from build123d import *

# Parameters (mm, degrees)
SKETCH1_W           = 50.8
SKETCH1_H           = 50.8
BOSS_EXTRUDE1_DEPTH = 2.54
SKETCH2_W           = 50.8
SKETCH2_H           = 50.8
SKETCH2_W_2         = 45.72
SKETCH2_H_2         = 22.86
BOSS_EXTRUDE2_DEPTH = 25.4
SKETCH3_W           = 50.8
SKETCH3_H           = 10.16
CUT_EXTRUDE1_DEPTH  = 25.4


with BuildPart() as part:
    # Sketch1 → Boss-Extrude1 (new body)
    with BuildSketch(Plane(origin=(0, 0, 0), x_dir=(1, 0, 0), z_dir=(0, 1, 0))):
        with Locations((25.4, 25.4)):
            Rectangle(SKETCH1_W, SKETCH1_H)
    extrude(amount=BOSS_EXTRUDE1_DEPTH)

    # Sketch2 → Boss-Extrude2 (add)
    with BuildSketch(Plane(origin=(0, 2.54, 0), x_dir=(1, 0, 0), z_dir=(0, 1, 0))):
        with Locations((25.4, 25.4)):
            Rectangle(SKETCH2_W, SKETCH2_H)
        with Locations((25.4, 25.4)):
            Rectangle(SKETCH2_W_2, SKETCH2_H_2, mode=Mode.SUBTRACT)
    extrude(amount=BOSS_EXTRUDE2_DEPTH)

    # Sketch3 → Cut-Extrude1 (cut)
    with BuildSketch(Plane(origin=(0, 27.94, 0), x_dir=(1, 0, 0), z_dir=(0, 1, 0))):
        with Locations((25.4, 45.72)):
            Rectangle(SKETCH3_W, SKETCH3_H)
        with Locations((25.4, 5.08)):
            Rectangle(SKETCH3_W, SKETCH3_H)
    extrude(amount=-CUT_EXTRUDE1_DEPTH, mode=Mode.SUBTRACT)


solid = part.part
CAD build for the part. Positions are in the model's coordinates, mm. A direction names the side the tool comes from. Round coordinates to 2 decimals unless told otherwise and drop trailing zeros. Write each loop counter-clockwise with the first axis right and the second up, starting at its lowest first coordinate (ties: lowest second). Pieces come first, ordered by that corner, then holes. Notation, with made-up numbers: M 27,47 L 43,47 A12 cw 43,63 Z; hole C 89.25,-12 d1. An arc over 180 degrees is marked long. Put each result on its own line as item: value. Start each with the question number.
1) 3-axis set-ups, long thin cutter, end or side, ignore diameter. For faces 4 (the flat face through (23, 27.94, -13)), 5 (the flat face through (25, 15, -10.16)), 6 (the flat face through (25, 15, -40.64)), 7 (the flat face through (25, 1, 0)), 8 (the flat face through (25, 15, -36.83)): which of +Z, -Z, +X, -X, +Y, -Y reach the whole face in a straight line?
2) Pin check, flat tips, straight feed: pin 1 Ø12.5 at (x, y) = (36.5, 19) entering from -Z; pin 2 Ø8 at (x, z) = (35, -3.5) entering from +Y; pin 3 Ø3 at (x, y) = (26, 14.5) entering from +Z. Stop position of each tip, or through.
3) Pull direction Z, two halves, no side cores. Call faces 1 (the flat face through (25, 2.54, -46)), 2 (the flat face through (25, 1, -50.8)), 3 (the flat face through (48.26, 15, -25)): pulls with the +Z half, pulls with the -Z half, needs draft (parallel to the pull), parting line crosses it, or undercut.
4) Drill centre lines: probe 1 along X at (y, z) = (6.5, -32.5); probe 2 along Z at (x, y) = (20, 19.75); probe 3 along Y at (x, z) = (21.5, -48). Where is each one in solid material? Low to high. Write a range as [from, to].
5) Saw through at D-D, the plane z = -6.5. Write the cut outline in (x, y), and give its area (3 significant figures).
6) Saw through at C-C, the plane y = 18.25. Write the cut outline in (x, z).
7) Saw through at A-A, the plane x = 30. Write the cut outline in (y, z).
8) Saw through at B-B, the plane z = -33. Write the cut outline in (x, y), and give its area (3 significant figures).
Resolved:
1. face 4: +Z, -Z, +X, -X, +Y
1. face 5: +Z, +X, -X, +Y
1. face 6: -Z, +X, -X, +Y
1. face 7: +Z, +X, -X, +Y, -Y
1. face 8: +Y
2. pin 1: z = -40.64
2. pin 2: y = 2.54
2. pin 3: z = -10.16
3. face 1: needs draft
3. face 2: pulls with the -Z half
3. face 3: undercut
4. probe 1: [0, 2.54], [48.26, 50.8]
4. probe 2: [-40.64, -36.83], [-13.97, -10.16]
4. probe 3: [0, 2.54]
5. outline: M 0,0 L 50.8,0 L 50.8,2.54 L 0,2.54 Z
5. area: 129 mm²
6. outline: M 0,-40.64 L 50.8,-40.64 L 50.8,-10.16 L 0,-10.16 Z; hole M 2.54,-36.83 L 48.26,-36.83 L 48.26,-13.97 L 2.54,-13.97 Z
7. outline: M 0,-50.8 L 2.54,-50.8 L 2.54,-40.64 L 27.94,-40.64 L 27.94,-36.83 L 2.54,-36.83 L 2.54,-13.97 L 27.94,-13.97 L 27.94,-10.16 L 2.54,-10.16 L 2.54,0 L 0,0 Z
8. outline: M 0,0 L 50.8,0 L 50.8,27.94 L 48.26,27.94 L 48.26,2.54 L 2.54,2.54 L 2.54,27.94 L 0,27.94 Z
8. area: 258 mm²
